For this review, take the finished solid that the model builds, in its own axes (mm). Round coordinates to 2 decimals unless told otherwise and drop trailing zeros. Order: outer loops, then holes, each group sorted by start corner. A loop starts at its lowest first (then second) coordinate and runs counter-clockwise, first axis right, second up. Notation, with made-up numbers: (50, 25) - (101, 25) arc R28 ccw to (101, 60) - close; hole circle Ø2 at (-10, 87). An arc over 180 degrees is marked (long way). One line per item, written item: value.
```python
from build123d import *

# Parameters (mm, degrees)
BOSS_EXTRUDE1_DEPTH = 30
SKETCH2_R           = 15
SKETCH2_R_2         = 5
CUT_EXTRUDE1_DEPTH  = 62.64414003


with BuildPart() as part:
    # Sketch1 → Boss-Extrude1 (new body)
    with BuildSketch(Plane.XY):
        with BuildLine():
            Line((-30, 20), (0, 20))
            ThreePointArc((0, 20), (20, 0), (0, -20))
            Line((0, -20), (-30, -20))
            ThreePointArc((-30, -20), (-50, 0), (-30, 20))
        make_face()
    extrude(amount=BOSS_EXTRUDE1_DEPTH)

    # Sketch2 → Cut-Extrude1 (cut, through all)
    with BuildSketch(Plane.XY):
        with Locations((-30, 0)):
            Circle(SKETCH2_R)
        Circle(SKETCH2_R_2)
    extrude(amount=CUT_EXTRUDE1_DEPTH, mode=Mode.SUBTRACT)


solid = part.part
```
Item 1: Take a section at C-C (z = 3.5). Write out the cut boundary in (x, y).
Returned:
outline: (-30, -20) - (0, -20) arc R20 ccw to (0, 20) - (-30, 20) arc R20 ccw to start; hole circle Ø30 at (-30, 0); hole circle Ø10 at (0, 0)
Item 2: Take a section at B-B (y = -6.5). Write out the cut boundary in (x, z), plus the area to 3 significant figures.
Returned:
outline: (-48.91, 0) - (-43.52, 0) - (-43.52, 30) - (-48.91, 30) - close; (-16.48, 0) - (18.91, 0) - (18.91, 30) - (-16.48, 30) - close
area: 1,220 mm^2
Item 3: Take a section at A-A (x = -38.5). Write out the cut boundary in (y, z).
Returned:
outline: (-18.1, 0) - (-12.36, 0) - (-12.36, 30) - (-18.1, 30) - close; (12.36, 0) - (18.1, 0) - (18.1, 30) - (12.36, 30) - close
Item 4: Take a section at D-D (x = 15.5). Write out the cut boundary in (y, z).
Returned:
outline: (-12.64, 0) - (12.64, 0) - (12.64, 30) - (-12.64, 30) - close
Item 5: For P1, Ø1.5, axis at x = 4.5, z = 19.5, coming from the -Y side; P2, Ø8, axis at y = -10, z = 20, coming from the -X side; P3, Ø10, axis at y = 8, z = 20, coming from the -X side, all flat-tipped, find the tip position at first contact; note any pin that passes through.
Returned:
P1: y = -19.65
P2: x = -49.08
P3: x = -49.77
Item 6: The part is to be moulded in two halves that separate along X. For faces 1 (the cylindrical face through (-1.08, -4.88, 14.79)), 2 (the flat face through (-15, 20, 15)), 3 (the cylindrical face through (-50, 0, 15)), 4 (the cylindrical face through (-44.985, 0.66, 14.79)), say which applies: +X half, -X half, draft (parallel to the pull), parting line (faces both ways), or undercut.
Returned:
face 1: undercut
face 2: draft
face 3: -X half
face 4: undercut
Item 7: Wall thickness on line 1 (Y direction, x = -30, z = 8.5); line 2 (X direction, y = 0, z = 9.5); line 3 (X direction, y = 2, z = 20.5): over which ranges is each line inside the solid? List them lowest first.
Returned:
line 1: -20 to -15, 15 to 20
line 2: -50 to -45, -15 to -5, 5 to 20
line 3: -49.9 to -44.87, -15.13 to -4.58, 4.58 to 19.9
